Could you check a few things on this model? Use its own coordinates, in mm. Face numbers are marked on the shaded views. A direction names the side the tool comes from. Give positions to 0.01 mm unless a question says otherwise; leave off trailing zeros. Write each loop counter-clockwise with the first axis right and the second up, starting at its lowest first coordinate (ties: lowest second). Pieces come first, ordered by that corner, then holes. Notation, with made-up numbers: (80.5, 52) - (94.5, 52) arc R25 ccw to (94.5, 69) - close; hole circle Ø6 at (-16, -32). An arc over 180 degrees is marked (long way). Use one line per item in the form item = value.
```python
from build123d import *

# Parameters (mm, degrees)
SKETCH1_R           = 109.6
SKETCH1_R_2         = 3.2125
SKETCH1_R_3         = 93.6
BOSS_EXTRUDE1_DEPTH = 6.7
SKETCH2_R           = 72
SKETCH2_R_2         = 36.2
SKETCH2_R_3         = 7
BOSS_EXTRUDE3_DEPTH = 6.7
FILLET1_R           = 10
FILLET2_R           = 5
CHAMFER1_SIZE       = 4
CHAMFER2_SIZE       = 0.8
FILLET7_R           = 2.5
FILLET8_R           = 2.5


with BuildPart() as part:
    # Sketch1 → Boss-Extrude1 (new body)
    with BuildSketch(Plane(origin=(0, 0, 0), x_dir=(1, 0, 0), z_dir=(0, 1, 0))):
        with Locations(Location((0, 0, 0), (0, 0, 270))):
            Circle(SKETCH1_R)
        with Locations(Location((0, 101.6, 0), (0, 0, 270))):
            Circle(SKETCH1_R_2, mode=Mode.SUBTRACT)
        with Locations(Location((0, 0, 0), (0, 0, 270))):
            Circle(SKETCH1_R_3, mode=Mode.SUBTRACT)
        with Locations(Location((50.8, 87.988181025, 0), (0, 0, 270))):
            Circle(SKETCH1_R_2, mode=Mode.SUBTRACT)
        with Locations(Location((87.988181025, 50.8, 0), (0, 0, 270))):
            Circle(SKETCH1_R_2, mode=Mode.SUBTRACT)
        with Locations(Location((101.6, 0, 0), (0, 0, 270))):
            Circle(SKETCH1_R_2, mode=Mode.SUBTRACT)
        with Locations(Location((87.988181025, -50.8, 0), (0, 0, 270))):
            Circle(SKETCH1_R_2, mode=Mode.SUBTRACT)
        with Locations(Location((50.8, -87.988181024, 0), (0, 0, 270))):
            Circle(SKETCH1_R_2, mode=Mode.SUBTRACT)
        with Locations(Location((0, -101.6, 0), (0, 0, 270))):
            Circle(SKETCH1_R_2, mode=Mode.SUBTRACT)
        with Locations(Location((-50.8, -87.988181025, 0), (0, 0, 270))):
            Circle(SKETCH1_R_2, mode=Mode.SUBTRACT)
        with Locations(Location((-87.988181024, -50.8, 0), (0, 0, 270))):
            Circle(SKETCH1_R_2, mode=Mode.SUBTRACT)
        with Locations(Location((-101.6, 0, 0), (0, 0, 270))):
            Circle(SKETCH1_R_2, mode=Mode.SUBTRACT)
        with Locations(Location((-87.988181024, 50.8, 0), (0, 0, 270))):
            Circle(SKETCH1_R_2, mode=Mode.SUBTRACT)
        with Locations(Location((-50.8, 87.988181024, 0), (0, 0, 270))):
            Circle(SKETCH1_R_2, mode=Mode.SUBTRACT)
    extrude(amount=BOSS_EXTRUDE1_DEPTH)



with BuildPart() as body_2:
    # Sketch2 → Boss-Extrude3 (new body)
    with BuildSketch(Plane(origin=(0, 17.95, 0), x_dir=(1, 0, 0), z_dir=(0, 1, 0))):
        with Locations(Location((0, 0, 0), (0, 0, 270))):
            Circle(SKETCH2_R)
        with Locations(Location((0, 0, 0), (0, 0, 270))):
            Circle(SKETCH2_R_2, mode=Mode.SUBTRACT)
        with Locations(Location((0, 57.15, 0), (0, 0, 270))):
            Circle(SKETCH2_R_3, mode=Mode.SUBTRACT)
        with Locations(Location((54.352879906, 17.660321229, 0), (0, 0, 270))):
            Circle(SKETCH2_R_3, mode=Mode.SUBTRACT)
        with Locations(Location((33.591927169, -46.235321229, 0), (0, 0, 270))):
            Circle(SKETCH2_R_3, mode=Mode.SUBTRACT)
        with Locations(Location((-33.591927169, -46.235321229, 0), (0, 0, 270))):
            Circle(SKETCH2_R_3, mode=Mode.SUBTRACT)
        with Locations(Location((-54.352879906, 17.660321229, 0), (0, 0, 270))):
            Circle(SKETCH2_R_3, mode=Mode.SUBTRACT)
    extrude(amount=-BOSS_EXTRUDE3_DEPTH)


with BuildPart() as part_1:
    add(part.part)

    add(body_2.part)  # Sweep3 merges body 2
    # Sweep3: sweep along a curve in space
    with BuildLine() as sweep3_path:
        ThreePointArc((0, 11.25, 72), (50.911688245, 11.25, 50.911688245), (72, 11.25, 0))
        ThreePointArc((72, 11.25, 0), (50.911688245, 11.25, -50.911688245), (0, 11.25, -72))
        ThreePointArc((0, 11.25, -72), (-50.911688245, 11.25, -50.911688245), (-72, 11.25, 0))
        ThreePointArc((-72, 11.25, 0), (-50.911688245, 11.25, 50.911688245), (0, 11.25, 72))
    # Sketch4 → Sweep3 (sweep)
    with BuildSketch(Plane.XY):
        Polygon((72, 17.95), (93.6, 6.7), (93.6, 0), (72, 11.25), align=None)
    sweep(path=sweep3_path.line)

    # Fillet1
    fillet1_edges = [part_1.edges().sort_by_distance(p)[0] for p in [
        (50.911688245, 17.95, 50.911688245),
    ]]
    fillet(fillet1_edges, radius=FILLET1_R)

    # Fillet2
    fillet2_edges = [part_1.edges().sort_by_distance(p)[0] for p in [
        (66.185194719, 6.7, 66.185194719),
    ]]
    fillet(fillet2_edges, radius=FILLET2_R)

    # Chamfer1
    chamfer1_edges = [part_1.edges().sort_by_distance(p)[0] for p in [
        (0, 11.25, -36.2),
    ]]
    chamfer(chamfer1_edges, length=CHAMFER1_SIZE)

    # Chamfer2
    chamfer2_edges = [part_1.edges().sort_by_distance(p)[0] for p in [
        (-54.352879906, 11.25, -24.660321229),
        (-33.591927169, 11.25, 39.235321229),
        (33.591927169, 11.25, 39.235321229),
        (54.352879906, 11.25, -24.660321229),
        (0, 11.25, -64.15),
    ]]
    chamfer(chamfer2_edges, length=CHAMFER2_SIZE)

    # Fillet7
    fillet7_edges = [part_1.edges().sort_by_distance(p)[0] for p in [
        (50.911688245, 11.25, -50.911688245),
    ]]
    fillet(fillet7_edges, radius=FILLET7_R)

    # Fillet8
    fillet8_edges = [part_1.edges().sort_by_distance(p)[0] for p in [
        (66.185194719, 0, -66.185194719),
    ]]
    fillet(fillet8_edges, radius=FILLET8_R)


solid = part_1.part
```
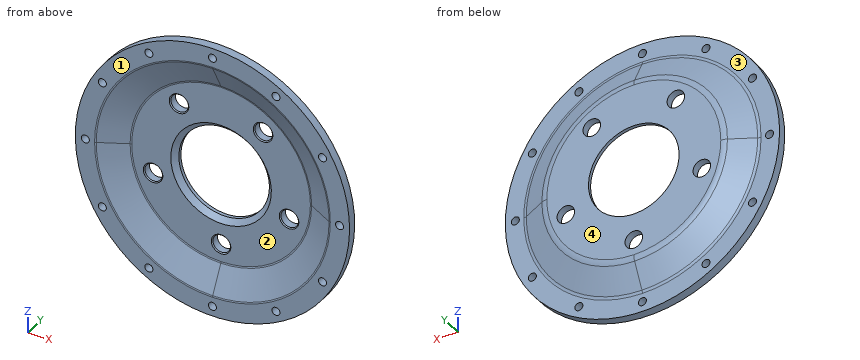
1. Imagine slicing it at B-B, the plane x = 101.6. List the corners of the cut face in (y, z) for me.
Response values:
outline = (0, -41.1) - (6.7, -41.1) - (6.7, -3.21) - (0, -3.21) - close; (0, 3.21) - (6.7, 3.21) - (6.7, 41.1) - (0, 41.1) - close
2. If I drill on line 1 (X direction, y = 5.25, z = 99); line 2 (Y direction, x = -16, z = 36); line 3 (X direction, y = 5.5, z = -38), over which ranges is the centre line in solid material (lowest first)? Write a range as from..to.
Response values:
line_1 = -47.02..-1.89, 1.89..47.02
line_2 = 12.05..17.95
line_3 = -102.8..-73.84, 73.84..102.8
3. For pin 1 (6 mm diameter, centred on y = 13, z = -7.5, fed in from +X); pin 2 (10.5 mm diameter, centred on x = 87.99, z = 50.8, fed in from +Y); pin 3 (6 mm diameter, centred on x = 62, z = -7, fed in from -Y); pin 4 (5 mm diameter, centred on x = -87.99, z = -50.8, fed in from +Y), each with a flat end and sliding along its axis, tell me the tip position at first contact or that it passes through.
Response values:
pin_1 = 86.95
pin_2 = 6.7
pin_3 = 11.25
pin_4 = through
4. Imagine slicing it at A-A, the plane z = -101.6. List the corners of the cut face in (x, y) for me.
Response values:
outline = (-41.1, 0) - (-3.21, 0) - (-3.21, 6.7) - (-41.1, 6.7) - close; (3.21, 0) - (41.1, 0) - (41.1, 6.7) - (3.21, 6.7) - close
5. Which directions (+Z, -Z, +X, -X, +Y, -Y) give clear straight access to the entire face, cutting with the end or side of a thin tool? Please do the marked faces 3 and 4.
Response values:
face_3 = +Y
face_4 = +Z, -Z, +X, -X, +Y
6. If we mould it in two halves opening along Z, with no side actions, what happens to the marked faces 1 and 2? For each: pulls with the +Z half, pulls with the -Z half, needs draft (parallel to the pull), parting line crosses it, or undercut.
Response values:
face_1 = needs draft
face_2 = undercut
7. Imagine slicing it at C-C, the plane z = -16. State how many separate pieces and enclosed holes the cut face has, and give its area (3 significant figures).
Response values:
separate_pieces = 4
enclosed_holes = 0
area = 816 mm²
